Verification items for the finished model (mm, model axes). A direction names the side the tool comes from. Give positions to 0.01 mm unless a question says otherwise; leave off trailing zeros. Order: outer loops, then holes, each group sorted by start corner. A loop starts at its lowest first (then second) coordinate and runs counter-clockwise, first axis right, second up. Notation, with made-up numbers: (50, -7) -> (108, -7) arc R10 cw to (108, -1) -> close; hole circle Ø7 at (38, 45.25). An arc over 180 degrees is marked (long way). Return JSON: item names as keys, results as strings. Group by question number.
(1) Cross-section at B-B on y = -10. Enter the section's corners in (x, z).
(2) Cross-section at C-C on y = 1.5. Enter the section's corners in (x, z).
(3) Thickness scan on line 1 along Y through (x, z) = (0.05, 2.5); line 2 along Z through (x, y) = (-1.2, -1.5); line 3 along X through (y, z) = (1, -0.7). Record the ranges inside material, lowest first.
(4) Tool access check on faces 1 (the face through (-0.521, 3.731, 2.347)), 2 (the face through (-2.45, 0.6, 0)). Record the directions out of +Z, -Z, +X, -X, +Y, -Y that give a thin tool (end or side, any length) a straight path to the whole face; none if there is none.
(5) Cross-section at A-A on y = -3.5. Enter the section's corners in (x, z) (3 decimals), then the cut area to 3 significant figures.
(6) Depth check by flat-ended pin: pin 1 Ø2 at (x, y) = (2, -10) entering from +Z; pin 2 Ø0.6 at (y, z) = (-1, 0) entering from -X; pin 3 Ø1.5 at (x, z) = (-1.5, 0) entering from -Y. Enter the tip coordinate at first touch or a pass-through.
from build123d import *

# Parameters (mm, degrees)
SKETCH1_R           = 2.75
BOSS_EXTRUDE1_DEPTH = 1.1
SKETCH2_R           = 2.45
DRAFT1_ANGLE        = 1
FILLET1_R           = 2.25
CUT_EXTRUDE1_DEPTH  = 1.1
SKETCH6_W           = 0.5
SKETCH6_H           = 0.5
BOSS_EXTRUDE2_DEPTH = 28
MOVE_FACE1_BY       = 1.6
SKETCH7_W           = 0.65
SKETCH7_H           = 1.25
BOSS_EXTRUDE3_DEPTH = 0.5
CHAMFER1_SIZE       = 0.05


with BuildPart() as part:
    # Sketch1 → Boss-Extrude1 (new body)
    with BuildSketch(Plane(origin=(0, 0, 0), x_dir=(1, 0, 0), z_dir=(0, 1, 0))):
        with Locations(Location((0, 0, 0), (0, 0, 270))):
            Circle(SKETCH1_R)
    extrude(amount=BOSS_EXTRUDE1_DEPTH)

    # Sweep1: sweep along a path in Sketch3
    with BuildLine(Plane.XY) as sweep1_path:
        Line((0, 1.1), (0, 8.5))
    # Sketch2 → Sweep1 (sweep)
    with BuildSketch(Plane(origin=(0, 1.1, 0), x_dir=(1, 0, 0), z_dir=(0, 1, 0))):
        Circle(SKETCH2_R)
    sweep(path=sweep1_path.line)

    # Draft1
    draft1_faces = [part.faces().sort_by_distance(p)[0] for p in [
        (-2.45, 4.8, 0),
    ]]
    draft(draft1_faces, Plane.ZX.offset(1.1), DRAFT1_ANGLE)

    # Fillet1
    fillet1_edges = [part.edges().sort_by_distance(p)[0] for p in [
        (-2.32083252, 8.5, 0),
    ]]
    fillet(fillet1_edges, radius=FILLET1_R)

    # Sketch5 → Cut-Extrude1 (cut)
    with BuildSketch(Plane(origin=(0, 1.1, 0), x_dir=(1, 0, 0), z_dir=(0, 1, 0))):
        with BuildLine():
            Line((-2.45, 1.2489996), (-2.45, -1.2489996))
            ThreePointArc((-2.45, -1.2489996), (-2.75, 0), (-2.45, 1.2489996))
        make_face()
    extrude(amount=-CUT_EXTRUDE1_DEPTH, mode=Mode.SUBTRACT)

    # Sketch6 → Boss-Extrude2 (add)
    with BuildSketch(Plane.XZ):
        with Locations((-1.27, 0)):
            Rectangle(SKETCH6_W, SKETCH6_H)
        with Locations((1.27, 0)):
            Rectangle(SKETCH6_W, SKETCH6_H)
    extrude(amount=BOSS_EXTRUDE2_DEPTH)

    # Move Face1: a face moved inward by 1.6
    extrude(part.faces().sort_by_distance((-1.27, -28, 0))[0], amount=MOVE_FACE1_BY, dir=(0, 1, 0), mode=Mode.SUBTRACT)

    # Sketch7 → Boss-Extrude3 (add)
    with BuildSketch(Plane.XY.offset(0.25)):
        with Locations((1.27, -3.625)):
            Rectangle(SKETCH7_W, SKETCH7_H)
        with Locations((-1.27, -3.625)):
            Rectangle(SKETCH7_W, SKETCH7_H)
    extrude(amount=-BOSS_EXTRUDE3_DEPTH)

    # Chamfer1
    chamfer1_edges = [part.edges().sort_by_distance(p)[0] for p in [
        (0.945, -3, 0),
        (1.595, -4.25, 0),
        (0.945, -4.25, 0),
        (1.595, -3, 0),
        (-1.595, -3, 0),
        (-0.945, -4.25, 0),
        (-1.595, -4.25, 0),
        (-0.945, -3, 0),
    ]]
    chamfer(chamfer1_edges, length=CHAMFER1_SIZE)


solid = part.part
Verdict:
{
 "1": {"outline": "(-1.52, -0.25) -> (-1.02, -0.25) -> (-1.02, 0.25) -> (-1.52, 0.25) -> close; (1.02, -0.25) -> (1.52, -0.25) -> (1.52, 0.25) -> (1.02, 0.25) -> close"},
 "2": {"outline": "circle Ø4.89 at (0, 0)"},
 "3": {"line 1": "0 to 1.1", "line 2": "-0.25 to 0.25", "line 3": "-2.45 to 2.66"},
 "4": {"face 1": "+Y", "face 2": "+Z, -Z, -X, +Y, -Y"},
 "5": {"outline": "(-1.595, -0.25) -> (-0.945, -0.25) -> (-0.945, 0.25) -> (-1.595, 0.25) -> close; (0.945, -0.25) -> (1.595, -0.25) -> (1.595, 0.25) -> (0.945, 0.25) -> close", "area": "0.650 mm²"},
 "6": {"pin 1": "z = 0.25", "pin 2": "x = -1.52", "pin 3": "y = -26.4"}
}
